Geometry: final body of the model. Coordinates: model frame, mm. Face numbers are marked on the shaded views. A direction names the side the tool comes from. Give positions to 0.01 mm unless a question says otherwise; leave off trailing zeros. Write each loop counter-clockwise with the first axis right and the second up, starting at its lowest first coordinate (ties: lowest second). Pieces come first, ordered by that corner, then holes. Notation, with made-up numbers: (-39.5, 26.5) - (-3.5, 26.5) arc R27 ccw to (-3.5, 50.5) - close; hole circle Ø11 at (42, -16.5). An arc over 180 degrees is marked (long way). Use CSV: the item, a comma, the result in double quotes. Start each with the question number.
(1) Reachability of the marked faces 1 and 2 from +Z, -Z, +X, -X, +Y, -Y: full face, straight path, thin tool, end or side. Return the list, or none.
(2) Section B-B on x = 60. Output: boundary loops of the cut face in (y, z), and give its area (3 significant figures).
(3) Section C-C on z = 110.5. Output: boundary loops of the cut face in (x, y), and give its area (3 significant figures).
(4) Line query: probe 1 along Z at (x, y) = (170, -6.25); probe 2 along Z at (x, y) = (-220, -7); probe 3 along X at (y, z) = (14.5, 10). Output: solid intervals per line, ascending. Write a range as [from, to].
(5) Section A-A on y = 59. Output: boundary loops of the cut face in (x, z).
(6) Draft query along X for the marked faces 3, 4 and 5. Return one class per face: released by +X, released by -X, zero draft, split by the parting line, or undercut.
(7) First-contact query: pin 1 Ø7 at (y, z) = (75, 0) entering from +X; pin 2 Ø14 at (y, z) = (75, 60) entering from -X; pin 3 Ø19 at (x, z) = (270, -26) entering from +Y. Flat tips, straight axial feed; report the tip coordinate or a pass-through.
from build123d import *

# Parameters (mm, degrees)
SKETCH1_W                       = 950
SKETCH1_H                       = 260
BASE_FLANGE1_DEPTH              = 10
EDGE_FLANGE1_STRIP_W            = 41.4732
EDGE_FLANGE1_STRIP_H            = 10
EDGE_FLANGE1_STRIP_CUT_DEPTH    = 260
EDGE_FLANGE1_STRIP_2_W          = 41.4732
EDGE_FLANGE1_STRIP_2_H          = 10
EDGE_FLANGE1_STRIP_CUT_2_DEPTH  = 260
EDGE_FLANGE1_DEPTH              = 260
EDGE_FLANGE1_BEND_DEPTH         = 260
BREAK_CORNER1_START             = -475
BREAK_CORNER1_DEPTH             = 950
M10_CLEARANCE_HOLE1_D           = 12
M10_CLEARANCE_HOLE1_CSINK_D     = 12.05
M10_CLEARANCE_HOLE1_CSINK_ANGLE = 90
M10_CLEARANCE_HOLE2_D           = 12
M10_CLEARANCE_HOLE2_CSINK_D     = 12.05
M10_CLEARANCE_HOLE2_CSINK_ANGLE = 90
FILLET1_R                       = 3


# Read off the part's stored shape, not the designer's step: Break-Corner1
# Sheet-metal steps are written as plain solids
with BuildPart() as part:
    # Sketch1 → Base-Flange1 (new body)
    with BuildSketch(Plane(origin=(0, 0, 0), x_dir=(1, 0, 0), z_dir=(0, 1, 0))):
        Rectangle(SKETCH1_W, SKETCH1_H)
    extrude(amount=-BASE_FLANGE1_DEPTH)

    # Edge-Flange1 strip (across the edge) → Edge-Flange1 strip cut (cut)
    with BuildSketch(Plane(origin=(-475, 0, -130), x_dir=(1, 0, 0), z_dir=(0, 0, 1))):
        with Locations((-10, -5)):
            Rectangle(EDGE_FLANGE1_STRIP_W, EDGE_FLANGE1_STRIP_H)
    extrude(amount=EDGE_FLANGE1_STRIP_CUT_DEPTH, mode=Mode.SUBTRACT)

    # Edge-Flange1 strip 2 (across the edge) → Edge-Flange1 strip cut 2 (cut)
    with BuildSketch(Plane(origin=(475, 0, 130), x_dir=(-1, 0, 0), z_dir=(0, 0, -1))):
        with Locations((-10, -5)):
            Rectangle(EDGE_FLANGE1_STRIP_2_W, EDGE_FLANGE1_STRIP_2_H)
    extrude(amount=EDGE_FLANGE1_STRIP_CUT_2_DEPTH, mode=Mode.SUBTRACT)

    # Edge-Flange1 section (across the edge) → Edge-Flange1 (add)
    with BuildSketch(Plane(origin=(-475, 0, -130), x_dir=(1, 0, 0), z_dir=(0, 0, 1))):
        with BuildLine():
            Line((0, 0.7366), (0, 105))
            Line((0, 105), (10, 105))
            Line((10, 105), (10, 0.7366))
            ThreePointArc((10, 0.7366), (10.215745145, 0.215745145), (10.7366, 0))
            Line((10.7366, 0), (10.7366, -10))
            ThreePointArc((10.7366, -10), (3.144677333, -6.855322667), (0, 0.7366))
        make_face()
    extrude(amount=EDGE_FLANGE1_DEPTH)

    # Edge-Flange1 section 2 (across the edge) → Edge-Flange1 bend (add)
    with BuildSketch(Plane(origin=(475, 0, 130), x_dir=(-1, 0, 0), z_dir=(0, 0, -1))):
        with BuildLine():
            Line((0, 0.7366), (0, 105))
            Line((0, 105), (10, 105))
            Line((10, 105), (10, 0.7366))
            ThreePointArc((10, 0.7366), (10.215745145, 0.215745145), (10.7366, 0))
            Line((10.7366, 0), (10.7366, -10))
            ThreePointArc((10.7366, -10), (3.144677333, -6.855322667), (0, 0.7366))
        make_face()
    extrude(amount=EDGE_FLANGE1_BEND_DEPTH)

    # Break-Corner1 outline → Break-Corner1 (cut)
    with BuildSketch(Plane.YZ.offset(BREAK_CORNER1_START)):
        Polygon((105, 130), (95, 130), (105, 120), align=None)
        Polygon((105, -130), (105, -120), (95, -130), align=None)
    extrude(amount=BREAK_CORNER1_DEPTH, mode=Mode.SUBTRACT)

    # M10 Clearance Hole1 (through all)
    with Locations(Plane(origin=(475, 0, 0), x_dir=(0, 0, -1), z_dir=(1, 0, 0))):
        with Locations((-90, 75), (-60, 75), (-30, 75), (0, 75), (30, 75), (60, 75), (90, 75)):
            CounterSinkHole(M10_CLEARANCE_HOLE1_D / 2, M10_CLEARANCE_HOLE1_CSINK_D / 2, counter_sink_angle=M10_CLEARANCE_HOLE1_CSINK_ANGLE)

    # M10 Clearance Hole2 (through all)
    with Locations(Plane(origin=(0, -10, 0), x_dir=(-1, 0, 0), z_dir=(0, -1, 0))):
        with Locations((-320, 78), (-220, 78), (-120, 78), (-270, 26), (-170, 26), (-270, -26), (-170, -26), (-320, -78), (-220, -78), (-120, -78)):
            m10_clearance_hole2 = CounterSinkHole(M10_CLEARANCE_HOLE2_D / 2, M10_CLEARANCE_HOLE2_CSINK_D / 2, counter_sink_angle=M10_CLEARANCE_HOLE2_CSINK_ANGLE)

    # Mirror1: M10 Clearance Hole2 across plane
    add(m10_clearance_hole2.mirror(Plane(origin=(0, 0, 0), x_dir=(0, 0, 1), z_dir=(1, 0, 0))), mode=Mode.SUBTRACT)

    # Fillet1
    fillet1_edges = [part.edges().sort_by_distance(p)[0] for p in [
        (465, 100, 125),
        (470, 105, 120),
        (475, 100, 125),
        (0, 0, 130),
        (0, -10, 130),
        (0, 0, -130),
        (0, -10, -130),
        (-471.855322667, -6.855322667, -130),
        (-471.855322667, -6.855322667, 130),
        (-464.784254855, 0.215745145, -130),
        (-464.784254855, 0.215745145, 130),
        (-465, 47.8683, 130),
        (-475, 47.8683, 130),
        (471.855322667, -6.855322667, 130),
        (471.855322667, -6.855322667, -130),
        (464.784254855, 0.215745145, 130),
        (464.784254855, 0.215745145, -130),
        (465, 47.8683, -130),
        (475, 47.8683, -130),
        (-465, 105, 0),
        (-475, 105, 0),
        (-470, 105, 120),
        (-465, 100, 125),
        (-470, 95, 130),
        (-475, 100, 125),
        (-475, 47.8683, -130),
        (-465, 47.8683, -130),
        (-470, 95, -130),
        (-465, 100, -125),
        (-470, 105, -120),
        (-475, 100, -125),
        (465, 105, 0),
        (475, 105, 0),
        (470, 105, -120),
        (465, 100, -125),
        (470, 95, -130),
        (475, 100, -125),
        (475, 47.8683, 130),
        (465, 47.8683, 130),
        (470, 95, 130),
    ]]
    fillet(fillet1_edges, radius=FILLET1_R)


solid = part.part
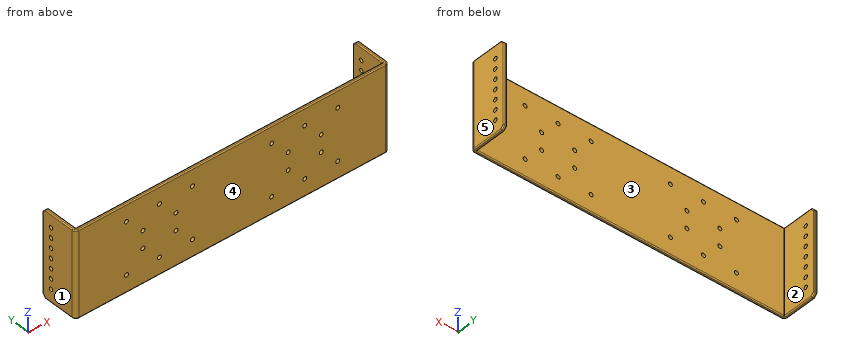
Check values:
1,face 1,"+Z, -Z, -X, +Y, -Y"
1,face 2,"+Z, -Z, +Y"
2,outline,"(-10, -127) arc R3 ccw to (-7, -130) - (-3, -130) arc R3 ccw to (0, -127) - (0, 127) arc R3 ccw to (-3, 130) - (-7, 130) arc R3 ccw to (-10, 127) - close"
2,area,"2,590 mm²"
3,outline,"(-475, 0.74) arc R10.74 ccw to (-464.26, -10) - (464.26, -10) arc R10.74 ccw to (475, 0.74) - (475, 102) arc R3 ccw to (472, 105) - (468, 105) arc R3 ccw to (465, 102) - (465, 0.74) arc R0.74 cw to (464.26, 0) - (-464.26, 0) arc R0.74 cw to (-465, 0.74) - (-465, 102) arc R3 ccw to (-468, 105) - (-472, 105) arc R3 ccw to (-475, 102) - close"
3,area,"11,500 mm²"
4,probe 1,"z = [-130, -32], [-20, 20], [32, 130]"
4,probe 2,"z = [-130, -84], [-72, 72], [84, 130]"
4,probe 3,"x = [-475, -465], [465, 475]"
5,outline,"(-475, -127) arc R3 ccw to (-472, -130) - (-468, -130) arc R3 ccw to (-465, -127) - (-465, 127) arc R3 ccw to (-468, 130) - (-472, 130) arc R3 ccw to (-475, 127) - close; (465, -127) arc R3 ccw to (468, -130) - (472, -130) arc R3 ccw to (475, -127) - (475, 127) arc R3 ccw to (472, 130) - (468, 130) arc R3 ccw to (465, 127) - close"
6,face 3,"undercut"
6,face 4,"zero draft"
6,face 5,"released by +X"
7,pin 1,"passes through"
7,pin 2,"stops at x = -475"
7,pin 3,"stops at y = 0"
